Job drawing, mm, ordinate dimensions from the low corner. One solid piece. Coordinates: 2 decimals unless noted, no trailing zeros. Loops run counter-clockwise (first coordinate to the right, second up) from the corner with the lowest first, then second, coordinate; pieces in that order, holes last. Notation, with made-up numbers: M 29,-6 L 66,-6 A4 cw 66,1 Z; hole C 68.25,75 d9. An arc over 180 degrees is marked long. Answer as a JSON object with one key per item and string values. Group by question number.
1. Saw through at B-B on z = 18. Write the cut outline in (x, y), then the cut area to 3 significant figures.
2. Drop flat-ended pins along their axis: pin 1 Ø6 at (x, z) = (17, 18) entering from -Y; pin 2 Ø2 at (y, z) = (5, 12) entering from -X. Give the stop position or say it passes through.
3. Drill centre lines: L1, parallel to Z at x = 18.75, y = 11.5; L2, parallel to Y at x = 22.5, z = 16.5; L3, parallel to Y at x = 22.75, z = 26. Where is each one in solid material? Low to high.
4. Saw through at A-A on y = 8.25. Write the cut outline in (x, z).
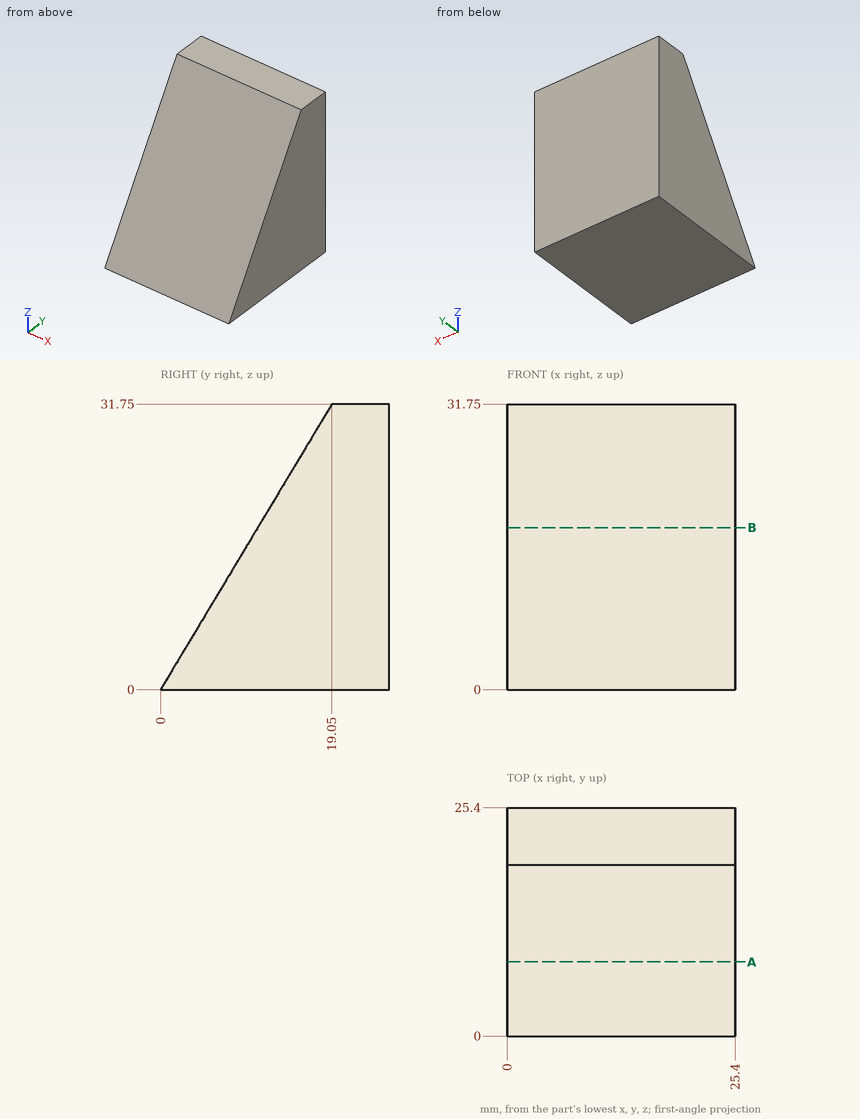
Outcome:
{
 "1": {"outline": "M 0,10.8 L 25.4,10.8 L 25.4,25.4 L 0,25.4 Z", "area": "371 mm²"},
 "2": {"pin 1": "stops at y = 9", "pin 2": "passes through"},
 "3": {"L1": "z = 0 to 19.17", "L2": "y = 9.9 to 25.4", "L3": "y = 15.6 to 25.4"},
 "4": {"outline": "M 0,0 L 25.4,0 L 25.4,13.75 L 0,13.75 Z"}
}
